For this review, take the finished solid that the model builds, in its own axes (mm). A direction names the side the tool comes from. Coordinates: 2 decimals unless noted, no trailing zeros. Write each loop counter-clockwise with the first axis right and the second up, starting at its lowest first coordinate (ties: lowest second). Pieces come first, ordered by that corner, then holes.
1) To check wall thickness, follow line 1 along X through (y, z) = (22.5, 2.65); line 2 along X through (y, z) = (35, 0.3); line 3 along Y through (x, z) = (-30.5, 2.15). State the ranges of each line that lie inside material, in increasing order.
2) We need section C-C on x = -17. Write out the cut boundary in (y, z), then the cut area to 3 significant figures.
3) We need section B-B on y = -11. Write out the cut boundary in (x, z).
4) For faces 5 (the face through (15, 44, 2)), 6 (the face through (-39.1, -36, 2)), 7 (the face through (0, -35, 2)), 8 (the face through (-40.6, 28, 2)), list the 3-axis set-ups (+Z, -Z, +X, -X, +Y, -Y) from which the entire face can be reached by the end or side of a thin tool; tool diameter is ignored.
5) Insertion check: P1, Ø2, axis at x = -42.5, z = 1.5, coming from the +Y side; P2, Ø2, axis at x = -16.5, z = 1.5, coming from the -Y side; P3, Ø2.5, axis at y = 44, z = 2.5, coming from the +X side. Each pin has a flat end and moves straight along its axis. Give the tip position at first contact, or say it passes through.
6) We need section A-A on x = 23.5. Write out the cut boundary in (y, z).
7) We need section D-D on z = 0.8. Give the number of separate pieces and of enclosed holes in the cut face, then the cut area to 3 significant figures.
8) Mouldability with a two-part tool opening along X and no side actions: class faces 1 (the face through (-50, -41, 2)), 2 (the face through (-15, 43, 2)), 3 (the face through (25, -14, 2)), 4 (the face through (40.6, 39, 2)) as pulls with the +X half, pulls with the -X half, needs draft (parallel to the pull), parting line crosses it, or undercut.
from build123d import *

# Parameters (mm, degrees)
BOSS_EXTRUDE1_DEPTH = 5
CUT_EXTRUDE1_DEPTH  = 5
CUT_EXTRUDE2_DEPTH  = 10


with BuildPart() as part:
    # Sketch1 → Boss-Extrude1 (new body)
    with BuildSketch(Plane.XY):
        Polygon((20.5, -41), (20.5, -35), (-20.5, -35), (-20.5, -41), (-55, -41), (-55, 41), (-15, 41), (-15, 46), (15, 46), (15, 41), (55, 41), (55, -41), align=None)
    extrude(amount=BOSS_EXTRUDE1_DEPTH)

    # Sketch2 → Cut-Extrude1 (cut)
    with BuildSketch(Plane(origin=(0, 0, 0), x_dir=(-1, 0, 0), z_dir=(0, 0, -1))):
        Polygon((-40.6, -38), (-40.6, -41), (-45, -41), (-45, -38), (-46.5, -38), (-46.5, -34.6), (-45, -34.6), (-45, -20.8), (-40.6, -20.8), (-40.6, -34.6), (-39.1, -34.6), (-39.1, -38), align=None)
        Polygon((45, -41), (45, -38), (46.5, -38), (46.5, -34.6), (45, -34.6), (45, -20.8), (40.6, -20.8), (40.6, -34.6), (39.1, -34.6), (39.1, -38), (40.6, -38), (40.6, -41), align=None)
        Polygon((40.6, 38), (40.6, 41), (45, 41), (45, 38), (46.5, 38), (46.5, 34.6), (45, 34.6), (45, 20.8), (40.6, 20.8), (40.6, 34.6), (39.1, 34.6), (39.1, 38), align=None)
        Polygon((-45, 41), (-45, 38), (-46.5, 38), (-46.5, 34.6), (-45, 34.6), (-45, 20.8), (-40.6, 20.8), (-40.6, 34.6), (-39.1, 34.6), (-39.1, 38), (-40.6, 38), (-40.6, 41), align=None)
    extrude(amount=-CUT_EXTRUDE1_DEPTH, mode=Mode.SUBTRACT)

    # Sketch3 → Cut-Extrude2 (cut)
    with BuildSketch(Plane(origin=(0, 0, 0), x_dir=(-1, 0, 0), z_dir=(0, 0, -1))):
        with BuildLine():
            Line((-14.6, -14), (-35, -14))
            ThreePointArc((-35, -14), (-38, -11), (-35, -8))
            Line((-35, -8), (-14.6, -8))
            ThreePointArc((-14.6, -8), (-11.6, -11), (-14.6, -14))
        make_face()
        with BuildLine():
            Line((14.6, -14), (35, -14))
            ThreePointArc((35, -14), (38, -11), (35, -8))
            Line((35, -8), (14.6, -8))
            ThreePointArc((14.6, -8), (11.6, -11), (14.6, -14))
        make_face()
    extrude(amount=-CUT_EXTRUDE2_DEPTH, mode=Mode.SUBTRACT)


solid = part.part
Result:
1. line 1: x = -55 to -45, -40.6 to 40.6, 45 to 55
1. line 2: x = -55 to -46.5, -39.1 to 39.1, 46.5 to 55
1. line 3: y = -41 to -14, -8 to 41
2. outline: (-35, 0) - (-14, 0) - (-14, 5) - (-35, 5) - close; (-8, 0) - (41, 0) - (41, 5) - (-8, 5) - close
2. area: 350 mm2
3. outline: (-55, 0) - (-38, 0) - (-38, 5) - (-55, 5) - close; (-11.6, 0) - (11.6, 0) - (11.6, 5) - (-11.6, 5) - close; (38, 0) - (55, 0) - (55, 5) - (38, 5) - close
4. face 5: +Z, -Z, +X, +Y
4. face 6: +Z, -Z
4. face 7: +Z, -Z, -Y
4. face 8: +Z, -Z, +Y
5. P1: stops at y = 20.8
5. P2: stops at y = -35
5. P3: stops at x = 15
6. outline: (-41, 0) - (-14, 0) - (-14, 5) - (-41, 5) - close; (-8, 0) - (41, 0) - (41, 5) - (-8, 5) - close
7. separate pieces: 1
7. enclosed holes: 2
7. area: 8,230 mm2
8. face 1: needs draft
8. face 2: pulls with the -X half
8. face 3: undercut
8. face 4: undercut
